Verification items for this drawing (mm, ordinates from the low corner). A direction names the side the tool comes from. Round coordinates to 2 decimals unless told otherwise and drop trailing zeros. Write each loop counter-clockwise with the first axis right and the second up, starting at its lowest first coordinate (ties: lowest second). Pieces come first, ordered by that corner, then holes.
Item 1: Cross-section at C-C (y = 30). Enter the section's corners in (x, z).
Item 2: Cross-section at A-A (z = 23). Enter the section's corners in (x, y).
Item 3: Access from +Z, -Z, +X, -X, +Y, -Y to the whole of each face (thin tool, end or side, straight path). Record for the marked faces 1, 2 and 3.
Item 4: Cross-section at D-D (z = 17.5). Enter the section's corners in (x, y).
Item 5: Cross-section at B-B (x = 12). Enter the section's corners in (y, z), then the cut area to 3 significant figures.
Item 6: Scan lines: probe 1 along Y at (x, z) = (26.5, 10); probe 2 along X at (y, z) = (34, 9.5); probe 3 along X at (y, z) = (10.5, 10). Record each from-to range of solid material in increasing order.
Item 7: Depth check by flat-ended pin: P1, Ø12, axis at x = 14, z = 14, coming from the +Y side; P2, Ø6, axis at y = 13.5, z = 17.5, coming from the -X side; P3, Ø16, axis at x = 23.5, z = 15.5, coming from the -Y side. Enter the tip coordinate at first touch or a pass-through.
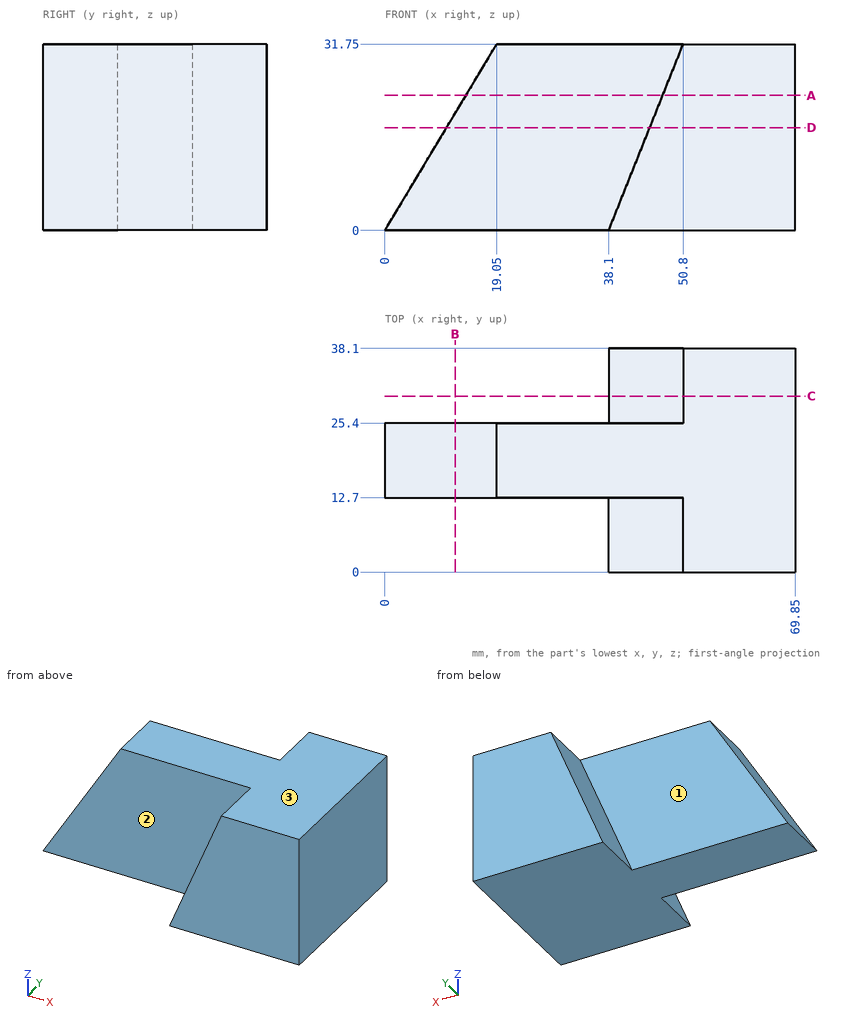
Resolved:
1. outline: (38.1, 0) - (69.85, 0) - (69.85, 31.75) - (50.8, 31.75) - close
2. outline: (13.8, 12.7) - (47.3, 12.7) - (47.3, 0) - (69.85, 0) - (69.85, 38.1) - (47.3, 38.1) - (47.3, 25.4) - (13.8, 25.4) - close
3. face 1: +Z, -X, +Y
3. face 2: +Z, -X, -Y
3. face 3: +Z, +X, -X, +Y, -Y
4. outline: (10.5, 12.7) - (45.1, 12.7) - (45.1, 0) - (69.85, 0) - (69.85, 38.1) - (45.1, 38.1) - (45.1, 25.4) - (10.5, 25.4) - close
5. outline: (12.7, 0) - (25.4, 0) - (25.4, 20) - (12.7, 20) - close
5. area: 254 mm2
6. probe 1: y = 12.7 to 25.4
6. probe 2: x = 41.9 to 69.85
6. probe 3: x = 42.1 to 69.85
7. P1: stops at y = 25.4
7. P2: stops at x = 8.7
7. P3: stops at y = 12.7
